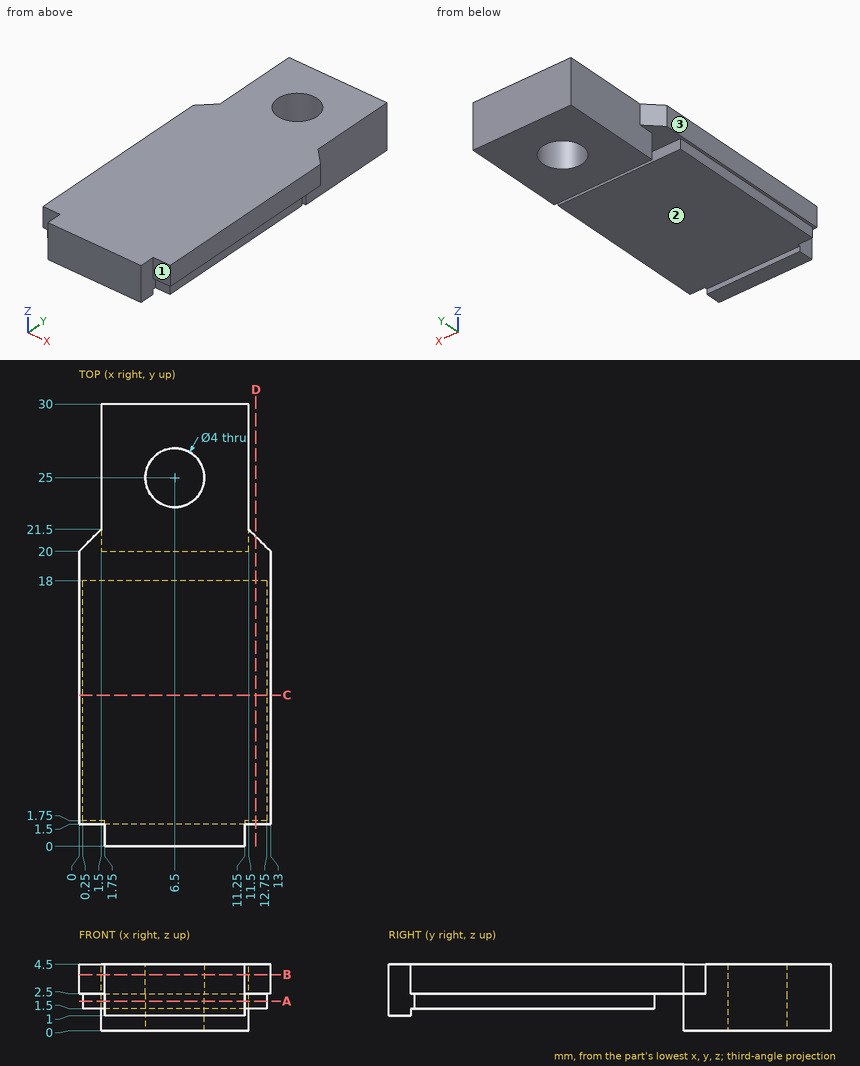
Geometry check sheet. Reference: drawing and pictorial views, mm from the part's lowest x, y, z. A direction names the side the tool comes from. Coordinates: 2 decimals unless noted, no trailing zeros. Loops run counter-clockwise (first coordinate to the right, second up) from the corner with the lowest first, then second, coordinate; pieces in that order, holes last. Notation, with made-up numbers: (66, 54) -> (120, 54) arc R20 cw to (120, 91) -> close; hole circle Ø3 at (-2, 0.5). An arc over 180 degrees is marked (long way). Write item = value, one per line. Start each with the question number.
1. Material ranges on line 1 (Y direction, x = 6.5, z = 1.25); line 2 (Y direction, x = 6.5, z = 2.15); line 3 (Y direction, x = 6.5, z = 3.05), recorded low to high.
2. Section check C-C on y = 10.25. Record the cut outline in (x, z), then the cut area to 3 significant figures.
3. Section check D-D on x = 12. Record the cut outline in (y, z).
4. Tool access check on the marked faces 1, 2 and 3. Record the directions out of +Z, -Z, +X, -X, +Y, -Y that give a thin tool (end or side, any length) a straight path to the whole face; none if there is none.
5. Section check A-A on z = 2. Record the cut outline in (x, y), then the cut area to 3 significant figures.
6. Depth check by flat-ended pin: P1, Ø0.8, axis at y = 8, z = 2, coming from the +X side; P2, Ø1.4, axis at x = 12, z = 3.5, coming from the -Y side; P3, Ø1.3, axis at y = 27.5, z = 2.5, coming from the +X side. Enter the tip coordinate at first touch or a pass-through.
7. Section check B-B on z = 3.8. Record the cut outline in (x, y).
Responses:
q1.line_1 = 0 to 1.5, 20 to 23, 27 to 30
q1.line_2 = 0 to 18, 20 to 23, 27 to 30
q1.line_3 = 0 to 23, 27 to 30
q2.outline = (0, 2.5) -> (0.25, 2.5) -> (0.25, 1.5) -> (12.75, 1.5) -> (12.75, 2.5) -> (13, 2.5) -> (13, 4.5) -> (0, 4.5) -> close
q2.area = 38.5 mm2
q3.outline = (1.5, 2.5) -> (1.75, 2.5) -> (1.75, 1.5) -> (18, 1.5) -> (18, 2.5) -> (21, 2.5) -> (21, 4.5) -> (1.5, 4.5) -> close
q4.face_1 = +Z, -Z, +X, -Y
q4.face_2 = -Z, +X, -X
q4.face_3 = +Z, -Z, -X, +Y, -Y
q5.outline = (0.25, 1.75) -> (1.75, 1.75) -> (1.75, 0) -> (11.25, 0) -> (11.25, 1.75) -> (12.75, 1.75) -> (12.75, 18) -> (0.25, 18) -> close; (1.5, 20) -> (11.5, 20) -> (11.5, 30) -> (1.5, 30) -> close; hole circle Ø4 at (6.5, 25)
q5.area = 307 mm2
q6.P1 = 12.75
q6.P2 = 1.5
q6.P3 = 11.5
q7.outline = (0, 1.5) -> (1.75, 1.5) -> (1.75, 0) -> (11.25, 0) -> (11.25, 1.5) -> (13, 1.5) -> (13, 20) -> (11.5, 21.5) -> (11.5, 30) -> (1.5, 30) -> (1.5, 21.5) -> (0, 20) -> close; hole circle Ø4 at (6.5, 25)
